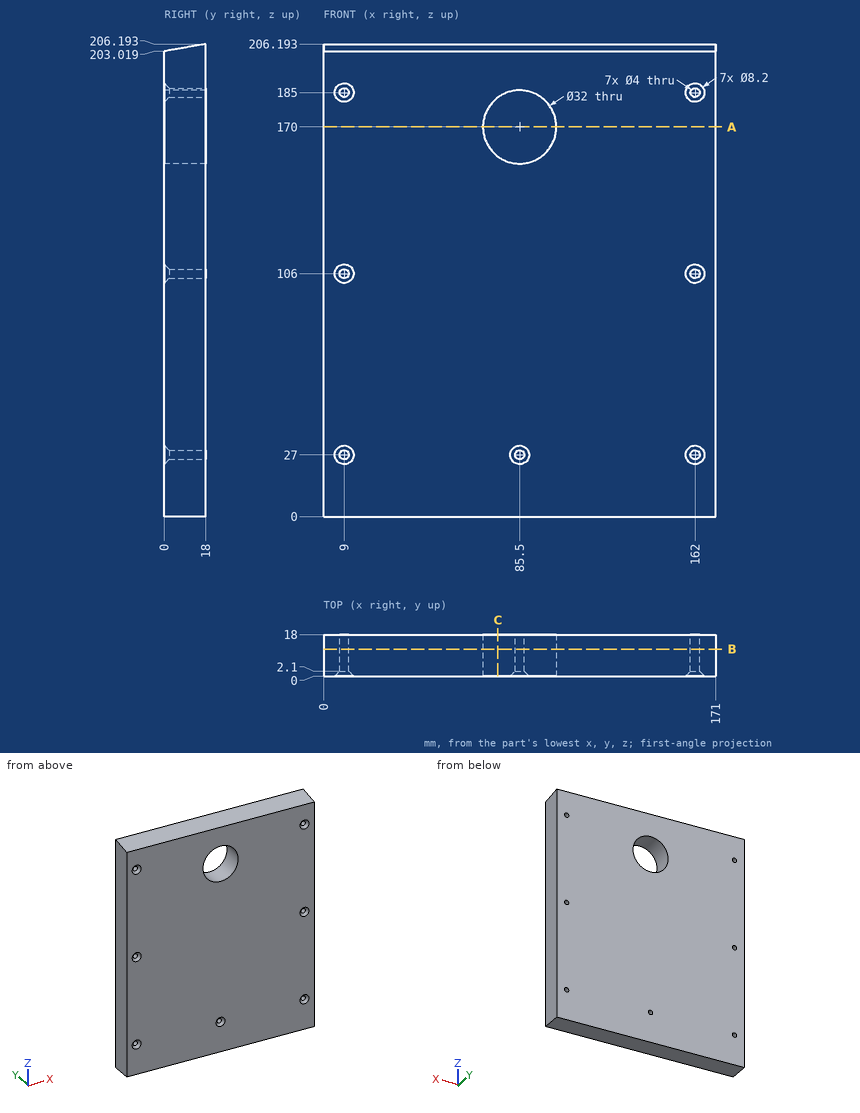
Study the drawing (mm; zero at the part's minimum x, y, z) and answer. Give positions to 0.01 mm unless a question says otherwise; leave off trailing zeros. Loops run counter-clockwise (first coordinate to the right, second up) from the corner with the lowest first, then second, coordinate; pieces in that order, holes last. Notation, with made-up numbers: (51, -25.75) -> (99, -25.75) arc R28 ccw to (99, 11.25) -> close; hole circle Ø9 at (71, 62). An arc over 180 degrees is marked (long way). Write item = value, one per line. Start each with the question number.
(1) Find the intervals of material crossed by probe 1 along X at (y, z) = (11.75, 27); probe 2 along Z at (x, y) = (85.5, 12) (3 decimals); probe 3 along Z at (x, y) = (9, 8), in increasing order. Write a range as from..to.
(2) Find section B-B on y = 11.75. Give the number of separate pieces and of enclosed holes in the cut face, and give its area (3 significant figures).
(3) Given pin 1 Ø3 at (x, y) = (122.5, 6.5) entering from +Z; pin 2 Ø4.5 at (x, z) = (162, 106) entering from +Y; pin 3 Ø1.5 at (x, y) = (58, 14) entering from +Z, each flat-ended and moving along its own axis, determine where each tip first touches the part or whether it passes through.
(4) Find section A-A on z = 170. Give the vertices of the cut face in (x, y), and give its area (3 significant figures).
(5) Find section C-C on x = 76. Give the vertices of the cut face in (y, z), and give its area (3 significant figures).
From the geometry:
q1.probe_1 = 0..7, 11..83.5, 87.5..160, 164..171
q1.probe_2 = 0..25, 29..154, 186..205.135
q1.probe_3 = 0..25, 29..104, 108..183, 187..204.43
q2.separate_pieces = 1
q2.enclosed_holes = 8
q2.area = 34,200 mm^2
q3.pin_1 = 204.43
q3.pin_2 = 18
q3.pin_3 = 205.62
q4.outline = (0, 0) -> (69.5, 0) -> (69.5, 18) -> (0, 18) -> close; (101.5, 0) -> (171, 0) -> (171, 18) -> (101.5, 18) -> close
q4.area = 2,500 mm^2
q5.outline = (0, 0) -> (18, 0) -> (18, 157.13) -> (0, 157.13) -> close; (0, 182.87) -> (18, 182.87) -> (18, 206.19) -> (0, 203.02) -> close
q5.area = 3,220 mm^2
